Check sheet for the modelled part. Datum: model origin and axes. Units: mm. Face numbers are marked on the shaded views. A direction names the side the tool comes from. Give positions to 0.01 mm unless a question says otherwise; leave off trailing zeros. Order: outer loops, then holes, each group sorted by start corner. A loop starts at its lowest first (then second) coordinate and runs counter-clockwise, first axis right, second up. Notation, with made-up numbers: (41.25, -12) - (99.25, -12) arc R7 cw to (99.25, -4) - close; hole circle Ø8 at (11.5, -40). An arc over 180 degrees is marked (long way). Answer in a Markdown table with one row per item.
from build123d import *

# Parameters (mm, degrees)
BOSS_EXTRUDE1_DEPTH = 3
SKETCH3_W           = 4.5
SKETCH3_H           = 5
BOSS_EXTRUDE2_DEPTH = 12
SKETCH4_W           = 5
SKETCH4_H           = 4
BOSS_EXTRUDE3_DEPTH = 12
SKETCH5_R           = 1.5
CUT_EXTRUDE1_DEPTH  = 12
SKETCH6_R           = 1.5
CUT_EXTRUDE2_DEPTH  = 12
SKETCH7_W           = 23
SKETCH7_H           = 5.5
BOSS_EXTRUDE5_DEPTH = 8
SKETCH8_W           = 2
SKETCH8_H           = 4.9
CUT_EXTRUDE3_DEPTH  = 28
FILLET1_R           = 2
SKETCH11_W          = 4
SKETCH11_H          = 12
BOSS_EXTRUDE6_DEPTH = 3.5
SKETCH12_W          = 2
SKETCH12_H          = 9
CUT_EXTRUDE5_DEPTH  = 10
FILLET3_R           = 2


with BuildPart() as part:
    # Sketch2 → Boss-Extrude1 (new body)
    with BuildSketch(Plane(origin=(0, 0, 0), x_dir=(1, 0, 0), z_dir=(0, 1, 0))):
        Polygon((-11.5, 5.5), (-11.5, -16.5), (11.5, -16.5), (11.5, 5.5), (16.5, 5.5), (16.5, 9.5), (11.5, 9.5), (11.5, 16.5), (-11.5, 16.5), (-11.5, 9.5), (-16.5, 9.5), (-16.5, 5.5), align=None)
    extrude(amount=BOSS_EXTRUDE1_DEPTH)

    # Sketch3 → Boss-Extrude2 (add)
    with BuildSketch(Plane.XZ):
        with Locations((-9.25, 14)):
            Rectangle(SKETCH3_W, SKETCH3_H)
        with Locations((-9.25, -14)):
            Rectangle(SKETCH3_W, SKETCH3_H)
    extrude(amount=BOSS_EXTRUDE2_DEPTH)

    # Sketch4 → Boss-Extrude3 (add)
    with BuildSketch(Plane(origin=(0, 3, 0), x_dir=(1, 0, 0), z_dir=(0, 1, 0))):
        with Locations((-14, 7.5)):
            Rectangle(SKETCH4_W, SKETCH4_H)
        with Locations((14, 7.5)):
            Rectangle(SKETCH4_W, SKETCH4_H)
    extrude(amount=BOSS_EXTRUDE3_DEPTH)

    # Sketch5 → Cut-Extrude1 (cut)
    with BuildSketch(Plane.XY.offset(-5.5)):
        with Locations((14, 9)):
            Circle(SKETCH5_R)
        with Locations((-14, 9)):
            Circle(SKETCH5_R)
    extrude(amount=-CUT_EXTRUDE1_DEPTH, mode=Mode.SUBTRACT)

    # Sketch6 → Cut-Extrude2 (cut)
    with BuildSketch(Plane(origin=(-7, 0, 0), x_dir=(0, 0, -1), z_dir=(1, 0, 0))):
        with Locations((-14, -6)):
            Circle(SKETCH6_R)
        with Locations((14, -6)):
            Circle(SKETCH6_R)
    extrude(amount=-CUT_EXTRUDE2_DEPTH, mode=Mode.SUBTRACT)

    # Sketch7 → Boss-Extrude5 (add)
    with BuildSketch(Plane(origin=(0, 3, 0), x_dir=(1, 0, 0), z_dir=(0, 1, 0))):
        with Locations((0, -17.25)):
            Rectangle(SKETCH7_W, SKETCH7_H)
    extrude(amount=BOSS_EXTRUDE5_DEPTH)

    # Sketch8 → Cut-Extrude3 (cut)
    with BuildSketch(Plane.ZY.offset(11.5)):
        with Locations((17.5, 7)):
            Rectangle(SKETCH8_W, SKETCH8_H)
    extrude(amount=-CUT_EXTRUDE3_DEPTH, mode=Mode.SUBTRACT)

    # Fillet1
    fillet1_edges = [part.edges().sort_by_distance(p)[0] for p in [
        (0, 3, 20),
        (0, 11, 20),
    ]]
    fillet(fillet1_edges, radius=FILLET1_R)

    # Sketch11 → Boss-Extrude6 (add)
    with BuildSketch(Plane(origin=(16.5, 0, 0), x_dir=(0, 0, -1), z_dir=(1, 0, 0))):
        with Locations((7.5, 9)):
            Rectangle(SKETCH11_W, SKETCH11_H)
    extrude(amount=BOSS_EXTRUDE6_DEPTH)

    # Sketch12 → Cut-Extrude5 (cut)
    with BuildSketch(Plane.XY.offset(-5.5)):
        with Locations((17.5, 9)):
            Rectangle(SKETCH12_W, SKETCH12_H)
    extrude(amount=-CUT_EXTRUDE5_DEPTH, mode=Mode.SUBTRACT)

    # Fillet3
    fillet3_edges = [part.edges().sort_by_distance(p)[0] for p in [
        (20, 3, -7.5),
        (20, 15, -7.5),
    ]]
    fillet(fillet3_edges, radius=FILLET3_R)


solid = part.part
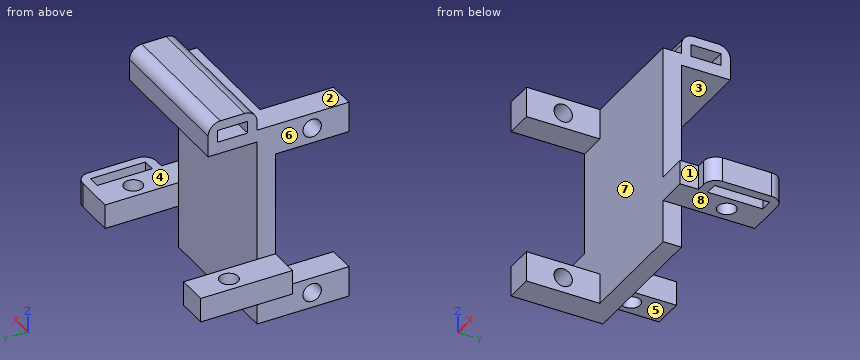
(1) Mould release check, pull along Z, two halves, no side actions. Record for the marked faces 6, 7 and 8: pulls with the +Z half, pulls with the -Z half, needs draft (parallel to the pull), parting line crosses it, or undercut.
Geometry says:
| item | result |
|---|---|
| face 6 | needs draft |
| face 7 | undercut |
| face 8 | pulls with the -Z half |
(2) Cross-section at A-A, the plane z = -14. Record the cut outline in (x, y).
Geometry says:
| item | result |
|---|---|
| outline | (-11.5, -12) - (-7, -12) - (-7, -7.5) - (-11.5, -7.5) - close; (-11.5, -4.5) - (-7, -4.5) - (-7, 0) - (11.5, 0) - (11.5, 3) - (-11.5, 3) - close |
(3) Gauge pin test, flat ends, axial feed: P1, Ø3, axis at x = -3.5, z = 16.5, coming from the +Y side; P2, Ø12, axis at x = -2, y = -8, coming from the +Z side; P3, Ø1.5, axis at y = 1, z = -12, coming from the +X side. Record the tip position at first contact, or that the pin passes through.
Geometry says:
| item | result |
|---|---|
| P1 | y = 11 |
| P2 | z = 16.5 |
| P3 | x = 11.5 |
(4) Cross-section at C-C, the plane y = -6. Record the cut outline in (x, z), then the cut area to 3 significant figures.
Geometry says:
| item | result |
|---|---|
| outline | (-11.5, -16.5) - (-7, -16.5) - (-7, -15.5) - (-11.5, -15.5) - close; (-11.5, -12.5) - (-7, -12.5) - (-7, -11.5) - (-11.5, -11.5) - close; (-11.5, 11.5) - (-7, 11.5) - (-7, 12.5) - (-11.5, 12.5) - close; (-11.5, 15.5) - (-7, 15.5) - (-7, 16.5) - (-11.5, 16.5) - close |
| area | 18.0 mm² |
(5) Access from +Z, -Z, +X, -X, +Y, -Y to the whole of each face (thin tool, end or side, straight path). Record for the marked faces 1, 2, 3, 4 and 5.
Geometry says:
| item | result |
|---|---|
| face 1 | +Z, -Z, +X, -Y |
| face 2 | +Z, +X, -X, -Y |
| face 3 | -Z, +X, -X, +Y |
| face 4 | +Z, +X, +Y, -Y |
| face 5 | -Z, -X, +Y, -Y |
(6) Cross-section at B-B, the plane y = 6.75. Record the cut outline in (x, z).
Geometry says:
| item | result |
|---|---|
| outline | (-16.5, -9.5) - (-11.5, -9.5) - (-11.5, -5.5) - (-16.5, -5.5) - close; (-11.5, 14.5) - (11.5, 14.5) - (11.5, 16.5) - (-11.5, 16.5) - close; (-11.5, 18.5) - (11.5, 18.5) - (11.5, 20) - (-11.5, 20) - close; (11.5, -9.5) - (16.5, -9.5) - (16.5, -5.5) - (11.5, -5.5) - close; (18.5, -9.5) - (20, -9.5) - (20, -5.5) - (18.5, -5.5) - close |
(7) Cross-section at D-D, the plane x = -14. Record the cut outline in (y, z), then the cut area to 3 significant figures.
Geometry says:
| item | result |
|---|---|
| outline | (0, -9.5) - (7.5, -9.5) - (7.5, -5.5) - (0, -5.5) - close; (10.5, -9.5) - (15, -9.5) - (15, -5.5) - (10.5, -5.5) - close |
| area | 48.0 mm² |
(8) Thickness scan on L1, parallel to Y at x = -9, z = -14; L2, parallel to Y at x = 14, z = -7; L3, parallel to Z at x = 9, y = 8.75. Record the ranges inside material, lowest first.
Geometry says:
| item | result |
|---|---|
| L1 | -12 to -7.5, -4.5 to 3 |
| L2 | 0 to 7.5, 10.5 to 15 |
| L3 | 14.5 to 16.5, 18.5 to 20 |
